```python
from build123d import *

# Parameters (mm, degrees)
F1_DEPTH     = 23
F2_R         = 0.325
F3_SIZE2     = 0.2309401077
F3_SIZE      = 0.4
F5_DEPTH     = 7
F7_DEPTH     = 1
F8_T1_DEPTH  = 2.6245000769
F8_T3_DEPTH  = 1.8050905296
F9_W         = 11.37
F9_H         = 1.5
F10_DEPTH    = 2
F11_R        = 0.325
F12_T1_DEPTH = 6.7216810245
F14_DEPTH    = 0.1
F15_W        = 1.2
F15_H        = 6.41
F15_H_2      = 7.41
F16_DEPTH    = 0.1
F17_T1_DEPTH = 15.6207881718


# Not quite as in the source:
# - a fillet or chamfer that OpenCascade refuses, or shapes differently, is made with other operations: its cross-section is extruded or revolved along the edge and cut away or added


with BuildPart() as f1:
    # F0 (on Front) → F1 (new body)
    with BuildSketch(Plane.XZ):
        Polygon((0, 1.92), (0, 0), (2.335, 0), (2.335, 1.5), (9.035, 1.5), (9.035, 0), (11.37, 0), (11.37, 1.92), align=None)
    extrude(amount=F1_DEPTH)

    # F2
    f2_edges = [f1.edges().sort_by_distance(p)[0] for p in [
        (11.37, -11.5, 0),
        (0, -11.5, 0),
    ]]
    fillet(f2_edges, radius=F2_R)

    # F3
    f3_edges = [f1.edges().sort_by_distance(p)[0] for p in [
        (5.685, -23, 1.92),
    ]]
    f3_side = f1.faces().sort_by_distance((5.685, -11.5, 1.92))[0]
    chamfer(f3_edges, length=F3_SIZE, length2=F3_SIZE2, reference=f3_side)

    # F4 (on Front) → F5 (join)
    with BuildSketch(Plane.XZ):
        with BuildLine():
            ThreePointArc((0, 0.325), (0.0951902961, 0.0951902961), (0.325, 0))
            Line((0.325, 0), (2.335, 0))
            Line((2.335, 0), (2.335, 1.9198597874))
            Line((2.335, 1.9198597874), (0, 1.92))
            Line((0, 1.92), (0, 0.325))
        make_face()
        with BuildLine():
            Line((9.035, 1.9067822723), (9.035, 0))
            Line((9.035, 0), (11.045, 0))
            ThreePointArc((11.045, 0), (11.2748097039, 0.0951902961), (11.37, 0.325))
            Line((11.37, 0.325), (11.37, 1.92))
            Line((11.37, 1.92), (9.035, 1.9067822723))
        make_face()
    extrude(amount=-F5_DEPTH)

    # F6 (on face) → F7 (join)
    with BuildSketch(Plane(origin=(0, 7, 0), x_dir=(-1, 0, 0), z_dir=(0, 1, 0))):
        with BuildLine():
            Line((-11.37, 0), (0, 0))
            Line((0, 0), (0, 4.5))
            ThreePointArc((0, 4.5), (-0.4145888759, 4.8120524944), (-0.8462680731, 5.1))
            Line((-0.8462680731, 5.1), (-10.5237319269, 5.1))
            ThreePointArc((-10.5237319269, 5.1), (-10.9554111241, 4.8120524944), (-11.37, 4.5))
            Line((-11.37, 4.5), (-11.37, 0))
        make_face()
    extrude(amount=-F7_DEPTH)

    # F8: fillet of radius 0.325 on 4 edges, made by hand

    # F8_s2 → F8_t1 (cut)
    with BuildSketch(Plane.XZ.offset(-7.8122500385)):
        with BuildLine():
            ThreePointArc((-0.0001, 0.3249), (0.0950902961, 0.0950902961), (0.3249, -0.0001))
            Line((0.3249, -0.0001), (0.3249, -0.0066))
            ThreePointArc((0.3249, -0.0066), (0.16245, -0.0065), (0, -0.0065))
            Line((0, -0.0065), (-0.0065, 0))
            ThreePointArc((-0.0065, 0), (-0.0065, 0.16245), (-0.0066, 0.3249))
            Line((-0.0066, 0.3249), (-0.0001, 0.3249))
        make_face()
        with BuildLine():
            ThreePointArc((11.3701, 0.3249), (11.2749097039, 0.0950902961), (11.0451, -0.0001))
            Line((11.0451, -0.0001), (11.0451, -0.0066))
            ThreePointArc((11.0451, -0.0066), (11.20755, -0.0065), (11.37, -0.0065))
            Line((11.37, -0.0065), (11.3765, 0))
            ThreePointArc((11.3765, 0), (11.3765, 0.16245), (11.3766, 0.3249))
            Line((11.3766, 0.3249), (11.3701, 0.3249))
        make_face()
    extrude(amount=F8_T1_DEPTH, mode=Mode.SUBTRACT)

    # F8_s4 → F8_t3 (cut)
    with BuildSketch(Plane.XZ.offset(-7.4025452648)):
        with BuildLine():
            ThreePointArc((-0.0001, 4.3418793672), (0.0333071199, 4.4854014639), (0.1266605677, 4.5994179613))
            Line((0.1266605677, 4.5994179613), (0.122695779, 4.6045687332))
            ThreePointArc((0.122695779, 4.6045687332), (0.0591315692, 4.5550650769), (-0.0040551807, 4.5050799123))
            Line((-0.0040551807, 4.5050799123), (-0.0065, 4.5))
            ThreePointArc((-0.0065, 4.5), (-0.0065, 4.4209396836), (-0.0066, 4.3418793672))
            Line((-0.0066, 4.3418793672), (-0.0001, 4.3418793672))
        make_face()
        with BuildLine():
            ThreePointArc((11.2433394323, 4.5994179613), (11.3366928801, 4.4854014639), (11.3701, 4.3418793672))
            Line((11.3701, 4.3418793672), (11.3766, 4.3418793672))
            ThreePointArc((11.3766, 4.3418793672), (11.3765, 4.4209396836), (11.3765, 4.5))
            Line((11.3765, 4.5), (11.3740551807, 4.5050799123))
            ThreePointArc((11.3740551807, 4.5050799123), (11.3108684308, 4.5550650769), (11.247304221, 4.6045687332))
            Line((11.247304221, 4.6045687332), (11.2433394323, 4.5994179613))
        make_face()
    extrude(amount=F8_T3_DEPTH, mode=Mode.SUBTRACT)

    # F9 (on face) → F10 (join)
    with BuildSketch(Plane.XY.offset(1.92)):
        with Locations((5.685, -13.6)):
            Rectangle(F9_W, F9_H)
    extrude(amount=F10_DEPTH)

    # F11
    f11_edges = [f1.edges().sort_by_distance(p)[0] for p in [
        (0, -13.6, 3.92),
        (11.37, -13.6, 3.92),
    ]]
    fillet(f11_edges, radius=F11_R)

    # F12: chamfer of 0.3 x 0.5196152423 on 2 edges, made by hand

    # F12_s2 → F12_t1 (cut)
    with BuildSketch(Plane.XY.offset(-1.0274508288)):
        Polygon((10.8503847577, 7), (11.37, 6.7), (11.37, 7), align=None)
        Polygon((0, 6.7), (0.5196152423, 7), (0, 7), align=None)
    extrude(amount=F12_T1_DEPTH, mode=Mode.SUBTRACT)

    # F13 (on face) → F14 (cut)
    with BuildSketch(Plane.XY.offset(1.92)):
        with BuildLine():
            Line((10.535, -14.35), (0.835, -14.35))
            Line((0.835, -14.35), (0.835, -21.35))
            ThreePointArc((0.835, -21.35), (0.9814466094, -21.7035533906), (1.335, -21.85))
            Line((1.335, -21.85), (10.035, -21.85))
            ThreePointArc((10.035, -21.85), (10.3885533906, -21.7035533906), (10.535, -21.35))
            Line((10.535, -21.35), (10.535, -14.35))
        make_face()
    extrude(amount=-F14_DEPTH, mode=Mode.SUBTRACT)

    # F15 (on face) → F16 (join, through all)
    with BuildSketch(Plane.XY.offset(1.82)):
        with Locations((4.585, -17.555)):
            Rectangle(F15_W, F15_H)
        with Locations((2.085, -18.055)):
            Rectangle(F15_W, F15_H_2)
        with Locations((9.285, -18.055)):
            Rectangle(F15_W, F15_H_2)
        with Locations((6.785, -17.555)):
            Rectangle(F15_W, F15_H)
    extrude(amount=F16_DEPTH)

    # F17: chamfer of 0.35 x 1.1447984165 on 1 edges, made by hand

    # F17_s2 → F17_t1 (cut)
    with BuildSketch(Plane.YZ.offset(-2.1253940859)):
        Polygon((6, 4.75), (7.1447984165, 5.1), (6, 5.1), align=None)
    extrude(amount=F17_T1_DEPTH, mode=Mode.SUBTRACT)


solid = f1.part
```
CAD build for the part. Positions are in the model's coordinates, mm. A direction names the side the tool comes from. Coordinates: 2 decimals unless noted, no trailing zeros. Write each loop counter-clockwise with the first axis right and the second up, starting at its lowest first coordinate (ties: lowest second). Pieces come first, ordered by that corner, then holes. Notation, with made-up numbers: (83, 4.5) -> (100, 4.5) arc R7 ccw to (100, 17.5) -> close; hole circle Ø10 at (31.25, 0.25). An arc over 180 degrees is marked (long way). Return JSON: item names as keys, results as strings. Group by question number.
Q1. Drill centre lines: line 1 (Y direction, x = 4.25, z = 3.5); line 2 (Z direction, x = 6, y = -8.75); line 3 (X direction, y = -9, z = 0.8) (3 decimals). Where is each one in solid material? Low to high.
Q2. Cut at B-B, the plane y = 2.25. Give the cut face in (x, z) (3 decimals).
Q3. Cut at C-C, the plane x = 4.75. Give the cut face in (y, z), then the cut area to 3 significant figures.
Q4. Which spindle directions (+Z, -Z, +X, -X, +Y, -Y) get a long thin tool onto all of the face, cutting with end or side? Do faces 5 (the face through (6, 6, 3)), 6 (the face through (9.4, -23, 0.9)), 7 (the face through (6, -6, 1.92)), 8 (the face through (6, -14, 3.92)), 9 (the face through (6, 7, 3)). Say none if no direction does.
Q5. Flat gauge pins, fed straight in: pin 1 (1.2 mm diameter, centred on x = 4.5, y = -13.5, fed in from +Z); pin 2 (0.7 mm diameter, centred on x = 1.5, y = 4.5, fed in from +Z); pin 3 (1.5 mm diameter, centred on x = 7.5, z = 4, fed in from -Y). Where does each tip first touch, or does it go through?
Q6. Pull direction X, two halves, no side cores. Call faces 1 (the face through (6, -18, 1.82)), 2 (the face through (5.7, -22.1, 1.92)), 3 (the face through (6, -11, 1.5)), 4 (the face through (0, -8, 1)): released by +X, released by -X, zero draft, split by the parting line, or undercut.
Q7. Cut at A-A, the plane z = 3.2. Give the cut face in (x, y), then the cut area to 3 significant figures.
Q8. Cut at D-D, the plane y = -4. Give the cut face in (x, z) (3 decimals).
Returned:
{
 "1": {"line 1": "y = -14.35 to -12.85, 6 to 7", "line 2": "z = 1.5 to 1.92", "line 3": "x = 0 to 2.335, 9.035 to 11.37"},
 "2": {"outline": "(0, 0.325) arc R0.325 ccw to (0.325, 0) -> (2.335, 0) -> (2.335, 1.92) -> (0, 1.92) -> close; (9.035, 0) -> (11.045, 0) arc R0.325 ccw to (11.37, 0.325) -> (11.37, 1.92) -> (9.035, 1.907) -> close"},
 "3": {"outline": "(-23, 1.5) -> (0, 1.5) -> (0, 1.92) -> (-12.85, 1.92) -> (-12.85, 3.92) -> (-14.35, 3.92) -> (-14.35, 1.92) -> (-20.76, 1.92) -> (-20.76, 1.82) -> (-21.85, 1.82) -> (-21.85, 1.92) -> (-22.6, 1.92) -> (-23, 1.69) -> close; (6, 0) -> (7, 0) -> (7, 5.06) -> (6, 4.75) -> close", "area": "17.4 mm2"},
 "4": {"face 5": "+Z", "face 6": "+Z, -Z, +X, -X, -Y", "face 7": "+Z, +X, -X", "face 8": "+Z, +X, -X, -Y", "face 9": "+Z, -Z, +X, -X, +Y"},
 "5": {"pin 1": "stops at z = 3.92", "pin 2": "stops at z = 1.92", "pin 3": "stops at y = -14.35"},
 "6": {"face 1": "undercut", "face 2": "zero draft", "face 3": "undercut", "face 4": "released by -X"},
 "7": {"outline": "(0, -14.35) -> (11.37, -14.35) -> (11.37, -12.85) -> (0, -12.85) -> close; (0, 6) -> (11.37, 6) -> (11.37, 6.7) -> (10.85, 7) -> (0.52, 7) -> (0, 6.7) -> close", "area": "28.3 mm2"},
 "8": {"outline": "(0, 0.325) arc R0.325 ccw to (0.325, 0) -> (2.335, 0) -> (2.335, 1.5) -> (9.035, 1.5) -> (9.035, 0) -> (11.045, 0) arc R0.325 ccw to (11.37, 0.325) -> (11.37, 1.92) -> (0, 1.92) -> close"}
}
